Check sheet for the modelled part. Datum: model origin and axes. Units: mm. A direction names the side the tool comes from. Coordinates: 2 decimals unless noted, no trailing zeros. Loops run counter-clockwise (first coordinate to the right, second up) from the corner with the lowest first, then second, coordinate; pieces in that order, holes last. Notation, with made-up numbers: (17, 88.25) -> (76, 88.25) arc R23 cw to (76, 125.25) -> close; hole circle Ø4 at (83.5, 6). An arc over 180 degrees is marked (long way). Use CSV: the item, a comma, the result in double quotes. Start each with the question number.
1. Release check for a two-part mould opening along Z. For faces 1 (the face through (-24, 12, 20)), 2 (the face through (20, 11, 0)), 3 (the face through (-78.1, 3.45, -17.34)), 4 (the face through (24, 12, -20)) record: pulls with the +Z half, pulls with the -Z half, needs draft (parallel to the pull), parting line crosses it, or undercut.
2. Set-up check for faces 5 (the face through (14.85, 2, 71.06)), 6 (the face through (-24, 12, -20)), 7 (the face through (24, 12, 20)), 8 (the face through (0, 4, -20)): record each of +Z, -Z, +X, -X, +Y, -Y from which the full face is reachable in a straight line by a thin tool's end or side.
3. Sectioned sample at C-C, the plane x = 7.5. Record the cut outline in (y, z), and give its area (3 significant figures).
4. Sectioned sample at D-D, the plane x = -35. Record the cut outline in (y, z), and give its area (3 significant figures).
5. Sectioned sample at B-B, the plane x = 75. Record the cut outline in (y, z).
6. Gauge pin test, flat ends, axial feed: pin 1 (1 mm diameter, centred on y = 8, z = -62.5, fed in from -X); pin 2 (8 mm diameter, centred on x = 36, y = 4.5, fed in from -Z); pin 3 (6.5 mm diameter, centred on x = -75, z = 0, fed in from -Y); pin 4 (7 mm diameter, centred on y = 14.5, z = 0, fed in from -X). Record the tip position at first contact, or that the pin passes through.
7. Sectioned sample at A-A, the plane y = 14.5. Record the cut outline in (x, z), and give its area (3 significant figures).
8. Thickness scan on L1, parallel to Y at x = 26, z = 0; L2, parallel to Y at x = 2, z = 27.5; L3, parallel to Z at x = 13, y = 3.25. Record the ranges inside material, lowest first.
```python
from build123d import *

# Parameters (mm, degrees)
SKETCH1_R               = 80
BOSS_EXTRUDE1_DEPTH     = 7
CUT_EXTRUDE1_REACH      = 115.353
SKETCH2_R               = 2.5
CUT_EXTRUDE2_REACH      = 115.353
SKETCH3_W               = 40
SKETCH3_H               = 40
SKETCH5_W               = 8
SKETCH5_H               = 40
BOSS_EXTRUDE2_DEPTH     = 15
FILLET1_SIZE            = 5
CUT_EXTRUDE4_REACH      = 138.191
SKETCH6_R               = 3
FILLET1_OF_MIRROR1_SIZE = 5
CUT_EXTRUDE3_REACH      = 116.127
SKETCH4_R               = 3
CUT_EXTRUDE5_START      = -2
CUT_EXTRUDE5_DEPTH      = 2
SKETCH8_R               = 12
CUT_EXTRUDE6_DEPTH      = 3


with BuildPart() as part:
    # Sketch1 → Boss-Extrude1 (new body)
    with BuildSketch(Plane(origin=(0, 0, 0), x_dir=(1, 0, 0), z_dir=(0, 1, 0))):
        with Locations(Location((0, 0, 0), (0, 0, 270))):
            Circle(SKETCH1_R)
    extrude(amount=BOSS_EXTRUDE1_DEPTH)

    # Sketch2 → Cut-Extrude1 (cut, up to next)
    with BuildSketch(Plane(origin=(0, 7, 0), x_dir=(1, 0, 0), z_dir=(0, 1, 0)), mode=Mode.PRIVATE) as cut_extrude1_sk1:
        with Locations(Location((-75, 0, 0), (0, 0, 270))):
            Circle(SKETCH2_R)
    cut_extrude1_tool1 = extrude(cut_extrude1_sk1.sketch, amount=-CUT_EXTRUDE1_REACH, mode=Mode.PRIVATE) & part.part
    # Sketch2 → Cut-Extrude1 (cut, up to next)
    with BuildSketch(Plane(origin=(0, 7, 0), x_dir=(1, 0, 0), z_dir=(0, 1, 0)), mode=Mode.PRIVATE) as cut_extrude1_sk2:
        with Locations(Location((0, 75, 0), (0, 0, 270))):
            Circle(SKETCH2_R)
    cut_extrude1_tool2 = extrude(cut_extrude1_sk2.sketch, amount=-CUT_EXTRUDE1_REACH, mode=Mode.PRIVATE) & part.part
    # Sketch2 → Cut-Extrude1 (cut, up to next)
    with BuildSketch(Plane(origin=(0, 7, 0), x_dir=(1, 0, 0), z_dir=(0, 1, 0)), mode=Mode.PRIVATE) as cut_extrude1_sk3:
        with Locations(Location((75, 0, 0), (0, 0, 270))):
            Circle(SKETCH2_R)
    cut_extrude1_tool3 = extrude(cut_extrude1_sk3.sketch, amount=-CUT_EXTRUDE1_REACH, mode=Mode.PRIVATE) & part.part
    add(cut_extrude1_tool1.solids().sort_by_distance((-75, 7, 0))[0], mode=Mode.SUBTRACT)
    add(cut_extrude1_tool2.solids().sort_by_distance((0, 7, -75))[0], mode=Mode.SUBTRACT)
    add(cut_extrude1_tool3.solids().sort_by_distance((75, 7, 0))[0], mode=Mode.SUBTRACT)

    # Sketch3 → Cut-Extrude2 (cut, up to next)
    with BuildSketch(Plane(origin=(0, 7, 0), x_dir=(1, 0, 0), z_dir=(0, 1, 0)), mode=Mode.PRIVATE) as cut_extrude2_sk1:
        Rectangle(SKETCH3_W, SKETCH3_H)
    cut_extrude2_tool1 = extrude(cut_extrude2_sk1.sketch, amount=-CUT_EXTRUDE2_REACH, mode=Mode.PRIVATE) & part.part
    add(cut_extrude2_tool1.solids().sort_by_distance((0, 7, 0))[0], mode=Mode.SUBTRACT)

    # Sketch5 → Boss-Extrude2 (add)
    with BuildSketch(Plane(origin=(0, 7, 0), x_dir=(1, 0, 0), z_dir=(0, 1, 0))):
        with Locations((-24, 0)):
            Rectangle(SKETCH5_W, SKETCH5_H)
    boss_extrude2 = extrude(amount=BOSS_EXTRUDE2_DEPTH)

    # Fillet1
    fillet1_edges = [part.edges().sort_by_distance(p)[0] for p in [
        (-24, 22, -20),
        (-24, 22, 20),
    ]]
    chamfer(fillet1_edges, length=FILLET1_SIZE)

    # Sketch6 → Cut-Extrude4 (cut, up to next)
    with BuildSketch(Plane.ZY.offset(28), mode=Mode.PRIVATE) as cut_extrude4_sk1:
        with Locations((0, 14.5)):
            Circle(SKETCH6_R)
    cut_extrude4_tool1 = extrude(cut_extrude4_sk1.sketch, amount=-CUT_EXTRUDE4_REACH, mode=Mode.PRIVATE) & part.part
    cut_extrude4 = cut_extrude4_tool1.solids().sort_by_distance((-28, 14.5, 0))[0]
    add(cut_extrude4, mode=Mode.SUBTRACT)

    # Mirror1: Boss-Extrude2, Cut-Extrude4 across plane
    add(boss_extrude2.mirror(Plane.ZY))
    add(cut_extrude4.mirror(Plane.ZY), mode=Mode.SUBTRACT)

    # Fillet1 of Mirror1
    fillet1_of_mirror1_edges = [part.edges().sort_by_distance(p)[0] for p in [
        (24, 22, -20),
        (24, 22, 20),
    ]]
    chamfer(fillet1_of_mirror1_edges, length=FILLET1_OF_MIRROR1_SIZE)

    # Sketch4 → Cut-Extrude3 (cut, up to next)
    with BuildSketch(Plane(origin=(0, 7, 0), x_dir=(1, 0, 0), z_dir=(0, 1, 0)), mode=Mode.PRIVATE) as cut_extrude3_sk1:
        with BuildLine():
            Line((-17, -37), (-17, -41))
            ThreePointArc((-17, -41), (-16, -42), (-15, -41))
            Line((-15, -41), (-15, -37))
            ThreePointArc((-15, -37), (-16, -36), (-17, -37))
        make_face()
    cut_extrude3_tool1 = extrude(cut_extrude3_sk1.sketch, amount=-CUT_EXTRUDE3_REACH, mode=Mode.PRIVATE) & part.part
    # Sketch4 → Cut-Extrude3 (cut, up to next)
    with BuildSketch(Plane(origin=(0, 7, 0), x_dir=(1, 0, 0), z_dir=(0, 1, 0)), mode=Mode.PRIVATE) as cut_extrude3_sk2:
        with BuildLine():
            Line((15, -37), (15, -41))
            ThreePointArc((15, -41), (16, -42), (17, -41))
            Line((17, -41), (17, -37))
            ThreePointArc((17, -37), (16, -36), (15, -37))
        make_face()
    cut_extrude3_tool2 = extrude(cut_extrude3_sk2.sketch, amount=-CUT_EXTRUDE3_REACH, mode=Mode.PRIVATE) & part.part
    # Sketch4 → Cut-Extrude3 (cut, up to next)
    with BuildSketch(Plane(origin=(0, 7, 0), x_dir=(1, 0, 0), z_dir=(0, 1, 0)), mode=Mode.PRIVATE) as cut_extrude3_sk3:
        with BuildLine():
            Line((15, -69), (15, -73))
            ThreePointArc((15, -73), (16, -74), (17, -73))
            Line((17, -73), (17, -69))
            ThreePointArc((17, -69), (16, -68), (15, -69))
        make_face()
    cut_extrude3_tool3 = extrude(cut_extrude3_sk3.sketch, amount=-CUT_EXTRUDE3_REACH, mode=Mode.PRIVATE) & part.part
    # Sketch4 → Cut-Extrude3 (cut, up to next)
    with BuildSketch(Plane(origin=(0, 7, 0), x_dir=(1, 0, 0), z_dir=(0, 1, 0)), mode=Mode.PRIVATE) as cut_extrude3_sk4:
        with BuildLine():
            Line((-17, -69), (-17, -73))
            ThreePointArc((-17, -73), (-16, -74), (-15, -73))
            Line((-15, -73), (-15, -69))
            ThreePointArc((-15, -69), (-16, -68), (-17, -69))
        make_face()
    cut_extrude3_tool4 = extrude(cut_extrude3_sk4.sketch, amount=-CUT_EXTRUDE3_REACH, mode=Mode.PRIVATE) & part.part
    # Sketch4 → Cut-Extrude3 (cut, up to next)
    with BuildSketch(Plane(origin=(0, 7, 0), x_dir=(1, 0, 0), z_dir=(0, 1, 0)), mode=Mode.PRIVATE) as cut_extrude3_sk5:
        with Locations(Location((0, -55, 0), (0, 0, 270))):
            Circle(SKETCH4_R)
    cut_extrude3_tool5 = extrude(cut_extrude3_sk5.sketch, amount=-CUT_EXTRUDE3_REACH, mode=Mode.PRIVATE) & part.part
    add(cut_extrude3_tool1.solids().sort_by_distance((-16, 7, 39))[0], mode=Mode.SUBTRACT)
    add(cut_extrude3_tool2.solids().sort_by_distance((16, 7, 39))[0], mode=Mode.SUBTRACT)
    add(cut_extrude3_tool3.solids().sort_by_distance((16, 7, 71))[0], mode=Mode.SUBTRACT)
    add(cut_extrude3_tool4.solids().sort_by_distance((-16, 7, 71))[0], mode=Mode.SUBTRACT)
    add(cut_extrude3_tool5.solids().sort_by_distance((0, 7, 55))[0], mode=Mode.SUBTRACT)

    # Sketch7 → Cut-Extrude5 (cut)
    # profile 1 of 4: a face of its own
    with BuildSketch(Plane.XZ.offset(CUT_EXTRUDE5_START)):
        with BuildLine():
            Line((-13.5, 69), (-13.5, 73))
            ThreePointArc((-13.5, 73), (-16, 75.5), (-18.5, 73))
            Line((-18.5, 73), (-18.5, 69))
            ThreePointArc((-18.5, 69), (-16, 66.5), (-13.5, 69))
        make_face()
        with BuildLine():
            ThreePointArc((-15, 69), (-16, 68), (-17, 69))
            Line((-17, 69), (-17, 73))
            ThreePointArc((-17, 73), (-16, 74), (-15, 73))
            Line((-15, 73), (-15, 69))
        make_face(mode=Mode.SUBTRACT)
    # profile 2 of 4: a face of its own
    with BuildSketch(Plane.XZ.offset(CUT_EXTRUDE5_START)):
        with BuildLine():
            Line((18.5, 69), (18.5, 73))
            ThreePointArc((18.5, 73), (16, 75.5), (13.5, 73))
            Line((13.5, 73), (13.5, 69))
            ThreePointArc((13.5, 69), (16, 66.5), (18.5, 69))
        make_face()
        with BuildLine():
            ThreePointArc((17, 69), (16, 68), (15, 69))
            Line((15, 69), (15, 73))
            ThreePointArc((15, 73), (16, 74), (17, 73))
            Line((17, 73), (17, 69))
        make_face(mode=Mode.SUBTRACT)
    # profile 3 of 4: a face of its own
    with BuildSketch(Plane.XZ.offset(CUT_EXTRUDE5_START)):
        with BuildLine():
            Line((-13.5, 37), (-13.5, 41))
            ThreePointArc((-13.5, 41), (-16, 43.5), (-18.5, 41))
            Line((-18.5, 41), (-18.5, 37))
            ThreePointArc((-18.5, 37), (-16, 34.5), (-13.5, 37))
        make_face()
        with BuildLine():
            ThreePointArc((-15, 37), (-16, 36), (-17, 37))
            Line((-17, 37), (-17, 41))
            ThreePointArc((-17, 41), (-16, 42), (-15, 41))
            Line((-15, 41), (-15, 37))
        make_face(mode=Mode.SUBTRACT)
    # profile 4 of 4: a face of its own
    with BuildSketch(Plane.XZ.offset(CUT_EXTRUDE5_START)):
        with BuildLine():
            Line((18.5, 37), (18.5, 41))
            ThreePointArc((18.5, 41), (16, 43.5), (13.5, 41))
            Line((13.5, 41), (13.5, 37))
            ThreePointArc((13.5, 37), (16, 34.5), (18.5, 37))
        make_face()
        with BuildLine():
            ThreePointArc((17, 37), (16, 36), (15, 37))
            Line((15, 37), (15, 41))
            ThreePointArc((15, 41), (16, 42), (17, 41))
            Line((17, 41), (17, 37))
        make_face(mode=Mode.SUBTRACT)
    extrude(amount=CUT_EXTRUDE5_DEPTH, mode=Mode.SUBTRACT)

    # Sketch8 → Cut-Extrude6 (cut)
    with BuildSketch(Plane(origin=(0, 7, 0), x_dir=(1, 0, 0), z_dir=(0, 1, 0))):
        with Locations(Location((0, -55, 0), (0, 0, 270))):
            Circle(SKETCH8_R)
    extrude(amount=-CUT_EXTRUDE6_DEPTH, mode=Mode.SUBTRACT)


solid = part.part
```
Completed:
1,face 1,"pulls with the +Z half"
1,face 2,"undercut"
1,face 3,"parting line crosses it"
1,face 4,"pulls with the -Z half"
2,face 5,"-Y"
2,face 6,"-Z, +X, -X, +Y"
2,face 7,"+Z, +X, -X, +Y"
2,face 8,"+Y, -Y"
3,outline,"(0, -79.65) -> (7, -79.65) -> (7, -20) -> (0, -20) -> close; (0, 20) -> (7, 20) -> (7, 45.63) -> (4, 45.63) -> (4, 64.37) -> (7, 64.37) -> (7, 79.65) -> (0, 79.65) -> close"
3,area,"779 mm²"
4,outline,"(0, -71.94) -> (7, -71.94) -> (7, 71.94) -> (0, 71.94) -> close"
4,area,"1,010 mm²"
5,outline,"(0, -27.84) -> (7, -27.84) -> (7, -2.5) -> (0, -2.5) -> close; (0, 2.5) -> (7, 2.5) -> (7, 27.84) -> (0, 27.84) -> close"
6,pin 1,"through"
6,pin 2,"z = -73.32"
6,pin 3,"y = 0"
6,pin 4,"x = -28"
7,outline,"(-28, -20) -> (-20, -20) -> (-20, -3) -> (-28, -3) -> close; (-28, 3) -> (-20, 3) -> (-20, 20) -> (-28, 20) -> close; (20, -20) -> (28, -20) -> (28, -3) -> (20, -3) -> close; (20, 3) -> (28, 3) -> (28, 20) -> (20, 20) -> close"
7,area,"544 mm²"
8,L1,"0 to 11.5, 17.5 to 22"
8,L2,"0 to 7"
8,L3,"-78.94 to -20, 20 to 78.94"
